Check sheet for the drawn part. Datum: minimum x, y, z corner. Units: mm. Give positions to 0.01 mm unless a question says otherwise; leave off trailing zeros. Write each loop counter-clockwise with the first axis right and the second up, starting at its lowest first coordinate (ties: lowest second). Pieces come first, ordered by that corner, then holes. Notation, with made-up numbers: (77, 12) - (112, 12) arc R6 cw to (112, 19) - close; hole circle Ø9 at (36.25, 89.25). An arc over 180 degrees is marked (long way). One line per question, with ' | ' between items. Start each with the question number.
Q1. Gauge pin test, flat ends, axial feed: P1, Ø8, axis at y = 11.5, z = 49.5, coming from the -X side; P2, Ø2, axis at x = 72, y = 6.5, coming from the -Z side; P3, Ø2, axis at x = 37.5, y = 9, coming from the -Z side. Record the tip position at first contact, or that the pin passes through.
Q2. Section check C-C on y = 11. Record the boundary of the cut face in (x, z).
Q3. Section check A-A on z = 45. Record the boundary of the cut face in (x, y), and give its area (3 significant figures).
Q4. Thickness scan on L1, parallel to Z at x = 45, y = 5; L2, parallel to Y at x = 83.5, z = 33.5. Record the ranges inside material, lowest first. Write a range as [from, to].
Q5. Release check for a two-part mould opening along Y. For the marked faces 1, 2 and 3 record: +Y half, -Y half, draft (parallel to the pull), parting line (faces both ways), or undercut.
Q6. Section check B-B on x = 45. Record the boundary of the cut face in (y, z), and give its area (3 significant figures).
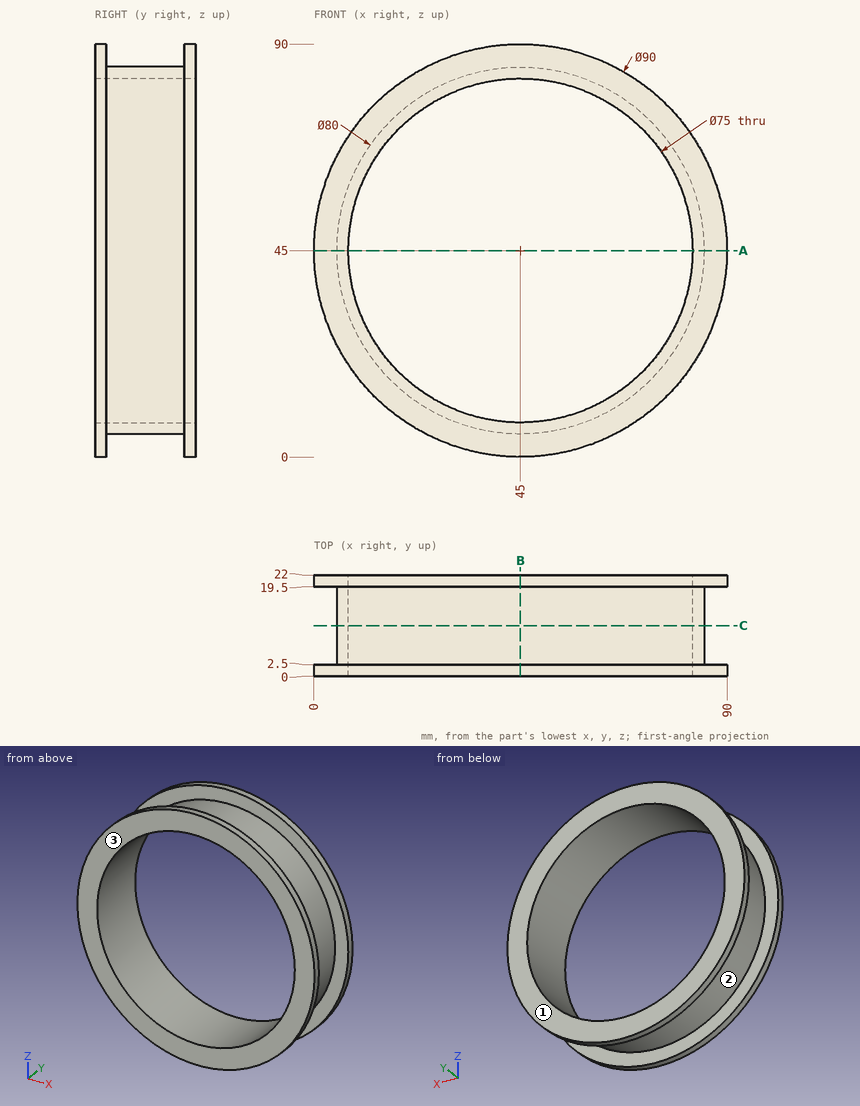
Working result:
1) P1: stops at x = 5 | P2: stops at z = 14.6 | P3: stops at z = 5.53
2) outline: circle Ø80 at (45, 45); hole circle Ø75 at (45, 45)
3) outline: (0, 0) - (7.5, 0) - (7.5, 22) - (0, 22) - (0, 19.5) - (5, 19.5) - (5, 2.5) - (0, 2.5) - close; (82.5, 0) - (90, 0) - (90, 2.5) - (85, 2.5) - (85, 19.5) - (90, 19.5) - (90, 22) - (82.5, 22) - close | area: 160 mm2
4) L1: z = [5, 7.5], [82.5, 85] | L2: y = [0, 2.5], [19.5, 22]
5) face 1: +Y half | face 2: undercut | face 3: -Y half
6) outline: (0, 0) - (2.5, 0) - (2.5, 5) - (19.5, 5) - (19.5, 0) - (22, 0) - (22, 7.5) - (0, 7.5) - close; (0, 82.5) - (22, 82.5) - (22, 90) - (19.5, 90) - (19.5, 85) - (2.5, 85) - (2.5, 90) - (0, 90) - close | area: 160 mm2
